Source: CAD feature listing. Evaluate the final solid. Frame: model axes, mm. Face numbers are marked on the shaded views. Give positions to 0.01 mm unless a question says otherwise; leave off trailing zeros. Loops run counter-clockwise (first coordinate to the right, second up) from the corner with the lowest first, then second, coordinate; pieces in that order, holes last. Notation, with made-up numbers: (13, 67.25) - (42, 67.25) arc R19 ccw to (42, 81.25) - close; hole circle Ø6 at (72, 75). An arc over 180 degrees is marked (long way). Put each result on its own line as item: value.
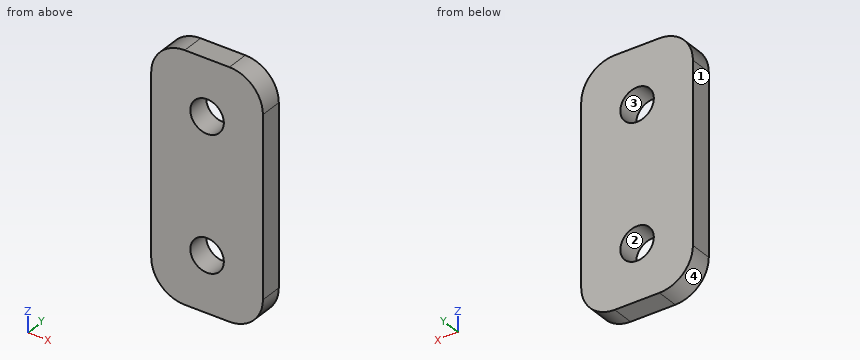
Autodesk Inventor part; units mm, degrees
ref_plane "YZ Plane" through (0, 0, 0) normal (1, 0, 0) x (0, 1, 0)
ref_plane "XZ Plane" through (0, 0, 0) normal (0, 1, 0) x (-1, 0, 0)
ref_plane "XY Plane" through (0, 0, 0) normal (0, 0, 1) x (1, 0, 0)
sketch "Sketch1" plane through (0, 0, 0) normal (0, 1, 0) x (-1, 0, 0)
  line L0 (1.5875, 0) -> (-2.17, 0) construction
  line L1 (0, 2.1822) -> (0, -1.8687) construction
  circle A0 centre (0, 6) radius 1.5
  line L2 (0, 11) -> (2, 11)
  line L3 (5, 8) -> (5, 0)
  arc A1 (5, 8) -> (2, 11) centre (2, 8) ccw
  line L4 (0, 11) -> (-2, 11)
  line L5 (-5, 8) -> (-5, 0)
  arc A2 (-2, 11) -> (-5, 8) centre (-2, 8) ccw
  circle A3 centre (0, -6) radius 1.5
  line L6 (0, -11) -> (2, -11)
  line L7 (5, -8) -> (5, 0)
  arc A4 (2, -11) -> (5, -8) centre (2, -8) ccw
  line L8 (-5, -8) -> (-5, 0)
  arc A5 (-5, -8) -> (-2, -11) centre (-2, -8) ccw
  line L9 (0, -11) -> (-2, -11)
  point P0 (0, 0)
  point P1 (5, 11)
  point P2 (-5, 11)
  point P3 (5, -11)
  point P4 (-5, -11)
  dimension "d0" = 3
  dimension "d1" = 6
  dimension "d2" = 5
  dimension "d3" = 5
  dimension "d4" = 3
extrude "Extrusion1" add sketch "Sketch1" along normal blind 2
properties part number "Konektor Casis 2_3DPrint"
1) Section query B-B, the plane x = 0. Output: boundary loops of the cut face in (y, z).
Check result:
outline: (0, -11) - (2, -11) - (2, -7.5) - (0, -7.5) - close; (0, -4.5) - (2, -4.5) - (2, 4.5) - (0, 4.5) - close; (0, 7.5) - (2, 7.5) - (2, 11) - (0, 11) - close
2) Section query C-C, the plane y = 1.55. Output: boundary loops of the cut face in (x, z).
Check result:
outline: (-5, -8) arc R3 ccw to (-2, -11) - (2, -11) arc R3 ccw to (5, -8) - (5, 8) arc R3 ccw to (2, 11) - (-2, 11) arc R3 ccw to (-5, 8) - close; hole circle Ø3 at (0, -6); hole circle Ø3 at (0, 6)
3) Section query D-D, the plane z = 6.5. Output: boundary loops of the cut face in (x, y).
Check result:
outline: (-5, 0) - (-1.41, 0) - (-1.41, 2) - (-5, 2) - close; (1.41, 0) - (5, 0) - (5, 2) - (1.41, 2) - close
4) Section query A-A, the plane z = -6. Output: boundary loops of the cut face in (x, y), plus the area to 3 significant figures.
Check result:
outline: (-5, 0) - (-1.5, 0) - (-1.5, 2) - (-5, 2) - close; (1.5, 0) - (5, 0) - (5, 2) - (1.5, 2) - close
area: 14.0 mm²
5) Mould query, pull axis Z, two halves, no side actions, for the marked faces 1, 2, 3 and 4. Classes: pulls with the +Z half, pulls with the -Z half, needs draft (parallel to the pull), parting line crosses it, or undercut.
Check result:
face 1: needs draft
face 2: undercut
face 3: undercut
face 4: pulls with the -Z half
6) Material intervals for line 1 along Z through (x, y) = (0, 1.25); line 2 along Z through (x, y) = (0.5, 1.25); line 3 along X through (y, z) = (1.7, 6.5), sorted ascending. Write a range as [from, to].
Check result:
line 1: [-11, -7.5], [-4.5, 4.5], [7.5, 11]
line 2: [-11, -7.41], [-4.59, 4.59], [7.41, 11]
line 3: [-5, -1.41], [1.41, 5]
